Job drawing, mm, ordinate dimensions from the low corner. One solid piece. A direction names the side the tool comes from. Give positions to 0.01 mm unless a question says otherwise; leave off trailing zeros. Loops run counter-clockwise (first coordinate to the right, second up) from the corner with the lowest first, then second, coordinate; pieces in that order, holes last. Notation, with made-up numbers: (7.5, 17) - (65.5, 17) arc R18 cw to (65.5, 32) - close; hole circle Ø10 at (75.5, -5). An arc over 180 degrees is marked (long way). Use a Markdown table: item, result.
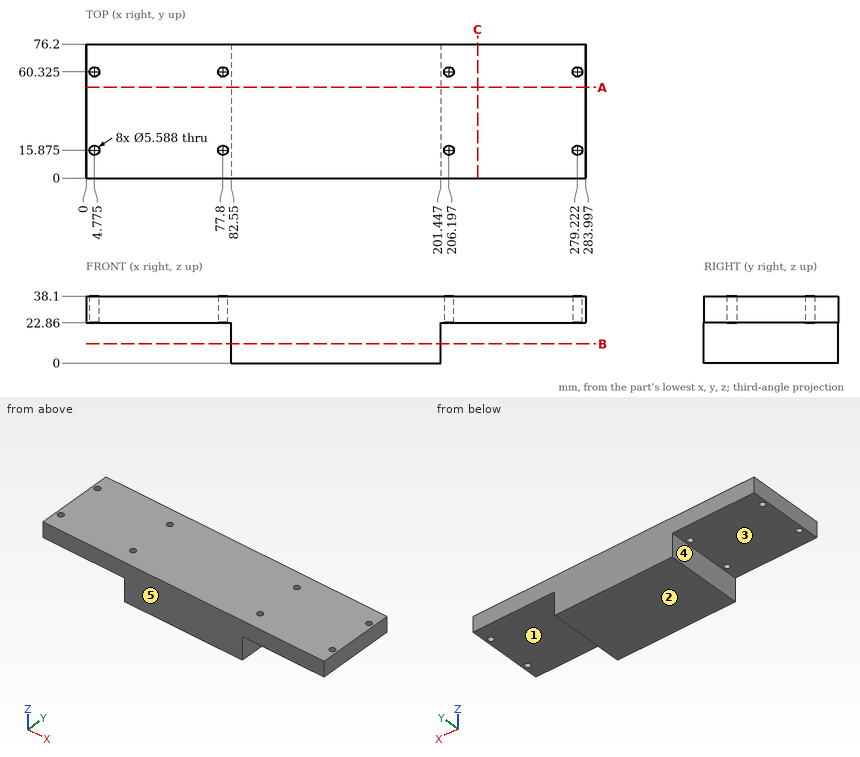
(1) Mould opens along X. For the marked faces 4 and 5 say: pulls with the +X half, pulls with the -X half, needs draft (parallel to the pull), parting line crosses it, or undercut.
Computed:
| item | result |
|---|---|
| face 4 | pulls with the -X half |
| face 5 | needs draft |
(2) Drill centre lines: probe 1 along Z at (x, y) = (262, 6); probe 2 along X at (y, z) = (18, 9). Where is each one in solid material? Low to high. Write a range as [from, to].
Computed:
| item | result |
|---|---|
| probe 1 | [22.86, 38.1] |
| probe 2 | [82.55, 201.45] |
(3) 3-axis set-ups, long thin cutter, end or side, ignore diameter. For the marked faces 1, 2 and 3: which of +Z, -Z, +X, -X, +Y, -Y reach the whole face in a straight line?
Computed:
| item | result |
|---|---|
| face 1 | -Z, +X, +Y, -Y |
| face 2 | -Z, +X, -X, +Y, -Y |
| face 3 | -Z, -X, +Y, -Y |
(4) Pin check, flat tips, straight feed: P1, Ø6.5, axis at x = 77.8, y = 60.32, coming from the -Z side; P2, Ø10, axis at y = 35, z = 9.5, coming from the +X side; P3, Ø7, axis at y = 52, z = 11, coming from the -X side. Stop position of each tip, or through.
Computed:
| item | result |
|---|---|
| P1 | z = 22.86 |
| P2 | x = 201.45 |
| P3 | x = 82.55 |
(5) Slice it at A-A, the plane y = 51.5. Write the cut outline in (x, z), plus the area to 3 significant figures.
Computed:
| item | result |
|---|---|
| outline | (0, 22.86) - (82.55, 22.86) - (82.55, 0) - (201.45, 0) - (201.45, 22.86) - (284, 22.86) - (284, 38.1) - (0, 38.1) - close |
| area | 7,050 mm² |
(6) Slice it at B-B, the plane z = 11. Write the cut outline in (x, y).
Computed:
| item | result |
|---|---|
| outline | (82.55, 0) - (201.45, 0) - (201.45, 76.2) - (82.55, 76.2) - close |
(7) Slice it at C-C, the plane x = 222.5. Write the cut outline in (y, z), plus the area to 3 significant figures.
Computed:
| item | result |
|---|---|
| outline | (0, 22.86) - (76.2, 22.86) - (76.2, 38.1) - (0, 38.1) - close |
| area | 1,160 mm² |
